```python
from build123d import *

# Parameters (mm, degrees)
SKETCH1_W          = 70
SKETCH1_H          = 3
CHAMFER1_SIZE      = 0.75
CUT_EXTRUDE2_DEPTH = 2.31


with BuildPart() as part:
    # Sketch1 → Revolve1 (revolve)
    with BuildSketch(Plane(origin=(0, 0, 0), x_dir=(0, 0, -1), z_dir=(1, 0, 0))):
        with Locations((35, 1.5)):
            Rectangle(SKETCH1_W, SKETCH1_H)
    revolve(axis=Axis((0, 0, -70), (0, 0, 1)))

    # Chamfer1
    chamfer1_edges = [part.edges().sort_by_distance(p)[0] for p in [
        (0, -3, -70),
    ]]
    chamfer(chamfer1_edges, length=CHAMFER1_SIZE)

    # Sketch7 → Revolve2 (revolve)
    with BuildSketch(Plane(origin=(0, 0, 0), x_dir=(0, 0, -1), z_dir=(1, 0, 0)), mode=Mode.PRIVATE) as revolve2_sk:
        Polygon((0, 6), (0.3, 6), (3.3, 3), (3.3, 0), (0, 0), align=None)
    revolve(revolve2_sk.sketch.rotate(Axis((0, 0, 0), (0, 0, -1)), 180), axis=Axis((0, 0, 0), (0, 0, -1)))

    # Boss-Extrude1 cone 1 section (through the dimple's axis) → Boss-Extrude1 (revolve)
    with BuildSketch(Plane(origin=(0, 0, -3.3), x_dir=(0, -1, 0), z_dir=(1, 0, 0))):
        Polygon((0, 0), (3, 0), (0, 3), align=None)
    revolve(axis=Axis((0, 0, -3.3), (0, 0, -1)))

    # Sketch5 → Cut-Extrude2 (cut)
    with BuildSketch(Plane.XY):
        Polygon((2, -1.154700538), (2, 1.154700538), (0, 2.309401077), (-2, 1.154700538), (-2, -1.154700538), (0, -2.309401077), align=None)
    extrude(amount=-CUT_EXTRUDE2_DEPTH, mode=Mode.SUBTRACT)

    # Cut-Extrude3 cone 1 section (through the dimple's axis) → Cut-Extrude3 (revolve, cut)
    with BuildSketch(Plane(origin=(0, 0, 0), x_dir=(0, -1, 0), z_dir=(1, 0, 0))):
        Polygon((0, 0), (2.309401077, 0), (0, 2.309401077), align=None)
    revolve(axis=Axis((0, 0, 0), (0, 0, -1)), mode=Mode.SUBTRACT)


solid = part.part
```
The listing builds one solid part. Answer for the finished solid, in the listing's coordinates (mm). A direction names the side the tool comes from. Coordinates: 2 decimals unless noted, no trailing zeros. Write each loop counter-clockwise with the first axis right and the second up, starting at its lowest first coordinate (ties: lowest second). Pieces come first, ordered by that corner, then holes. Notation, with made-up numbers: (1, -8) - (34, -8) arc R24 cw to (34, 2) - close; hole circle Ø4 at (-7, 54.5). An arc over 180 degrees is marked (long way). Return JSON: item names as keys, results as strings. Group by question number.
1. A cutting plane is placed at A-A, the plane y = 0. Determine the outline of the cut face in (x, z).
2. Determine the mould class of faces 1 (the conical face through (1.06, 1.87, -0.16)), 2 (the flat face through (0, 0, -70)), 3 (the cylindrical face through (0, -3, -37)) for opening direction Y: released by +Y, released by -Y, zero draft, split by the parting line, or undercut.
3. Given pin 1 (6 mm diameter, centred on y = 1, z = -61, fed in from +X); pin 2 (1.2 mm diameter, centred on y = 0, z = -1, fed in from +X); pin 3 (6 mm diameter, centred on y = 3, z = -38, fed in from -X); pin 4 (1.5 mm diameter, centred on x = 4.5, z = -23.5, fed in from -Y), each flat-ended and moving along its own axis, determine where each tip first touches the part or whether it passes through.
4. A cutting plane is placed at B-B, the plane z = -5.5. Determine the outline of the cut face in (x, y).
5. Which of the six approach directions +Z, -Z, +X, -X, +Y, -Y give full straight-line access (tool end or side, diameter ignored) to faces 4 (the conical face through (2.791, -1.452, -3.154)), 5 (the flat face through (-1.014, -1.724, -1.139))?
6. Straight lines are drawn through the part: L1, parallel to X at y = -2, z = -24.5; L2, parallel to Z at x = 0, y = 0.25; L3, parallel to Y at x = 0, z = -55. For each, find the intervals that lie inside material, in ascending order.
Ans:
{
 "1": {"outline": "(-6, -0.3) - (-3, -3.3) - (-3, -69.25) - (-2.25, -70) - (2.25, -70) - (3, -69.25) - (3, -3.3) - (6, -0.3) - (6, 0) - (2.31, 0) - (2, -0.31) - (2, -2.31) - (-2, -2.31) - (-2, -0.31) - (-2.31, 0) - (-6, 0) - close"},
 "2": {"face 1": "undercut", "face 2": "zero draft", "face 3": "split by the parting line"},
 "3": {"pin 1": "x = 3", "pin 2": "x = 5.9", "pin 3": "x = -3", "pin 4": "through"},
 "4": {"outline": "circle Ø6 at (0, 0)"},
 "5": {"face 4": "-Z", "face 5": "+Z"},
 "6": {"L1": "-2.24 to 2.24", "L2": "-70 to -2.31", "L3": "-3 to 3"}
}
